Autodesk Inventor part; units mm, degrees
ref_plane "YZ Plane" through (0, 0, 0) normal (1, 0, 0) x (0, 1, 0)
ref_plane "XZ Plane" through (0, 0, 0) normal (0, 1, 0) x (-1, 0, 0)
ref_plane "XY Plane" through (0, 0, 0) normal (0, 0, 1) x (1, 0, 0)
sketch "Sketch1" plane through (0, 0, 0) normal (0, 0, 1) x (1, 0, 0)
  line L0 (0, 0) -> (170, 0)
  line L1 (170, 0) -> (170, 170)
  line L2 (170, 170) -> (0, 170)
  line L3 (0, 170) -> (0, 0)
  dimension "d0" = 170
  dimension "d1" = 170
extrude "Extrusion1" add sketch "Sketch1" along normal blind 2
sketch "Sketch2" plane through (0, 0, 2) normal (0, 0, 1) x (1, 0, 0)
  line L0 (170, 170) -> (0, 170)
  line L1 (0, 170) -> (0, 0)
  line L2 (0, 170) -> (0, 159.84) construction
  line L3 (0, 159.84) -> (6.35, 159.84) construction
  line L4 (6.35, 170) -> (163.83, 170) construction
  line L5 (163.83, 170) -> (163.83, 136.98) construction
  line L6 (6.35, 159.84) -> (6.35, 4.9) construction
  line L7 (6.35, 4.9) -> (163.83, 4.9) construction
  circle A0 centre (6.35, 159.84) radius 1.98
  circle A1 centre (163.83, 136.98) radius 1.98
  circle A2 centre (6.35, 4.9) radius 1.98
  circle A3 centre (163.83, 4.9) radius 1.98
  dimension "d4" = 10.16
  dimension "d5" = 6.35
  dimension "d6" = 157.48
  dimension "d7" = 33.02
  dimension "d8" = 154.94
  dimension "d9" = 3.96
  dimension "d10" = 3.96
  dimension "d11" = 3.96
  dimension "d12" = 3.96
extrude "Extrusion2" cut sketch "Sketch2" against normal blind 2
sketch "Sketch3" plane through (0, 0, 2) normal (0, 0, 1) x (1, 0, 0)
  line L0 (14.2327, 124.8626) -> (6.35, 124.8626)
  line L1 (6.35, 124.8626) -> (6.35, 41.7782)
  line L2 (6.35, 41.7782) -> (14.2327, 41.7782)
  line L3 (14.2327, 41.7782) -> (14.2327, 124.8626)
extrude "Extrusion3" add sketch "Sketch3" along normal blind 2
sketch "Sketch4" plane through (0, 0, 4) normal (0, 0, 1) x (1, 0, 0)
  line L0 (14.2327, 124.8626) -> (6.35, 124.8626)
  line L1 (6.35, 124.8626) -> (6.35, 41.7782)
  line L2 (6.35, 41.7782) -> (14.2327, 41.7782)
  line L3 (14.2327, 41.7782) -> (14.2327, 124.8626)
  line L4 (12.3491, 93.2345) -> (12.3491, 74.2867) construction
  line L5 (12.3491, 74.2867) -> (8.2093, 74.2867) construction
  line L6 (8.2093, 74.2867) -> (8.2093, 93.2345) construction
  line L7 (8.2093, 93.2345) -> (12.3491, 93.2345) construction
  point P0 (0, 0)
sketch "Sketch5" plane through (0, 0, 2) normal (0, 0, 1) x (1, 0, 0)
  line L0 (170, 170) -> (0, 170)
  line L1 (17.1297, 170) -> (152.7432, 170)
  line L2 (152.7432, 170) -> (152.7432, 149.8199)
  line L3 (152.7432, 149.8199) -> (17.1297, 149.8199)
  line L4 (17.1297, 149.8199) -> (17.1297, 170)
extrude "Extrusion4" add sketch "Sketch5" along normal blind 2
sketch "Sketch6" plane through (0, 0, 4) normal (0, 0, 1) x (1, 0, 0)
  line L0 (17.1297, 170) -> (17.1297, 149.8199)
  line L1 (17.1297, 149.8199) -> (152.7432, 149.8199)
  line L2 (152.7432, 149.8199) -> (152.7432, 170)
  line L3 (152.7432, 170) -> (17.1297, 170)
  line L4 (74.7193, 163.8007) -> (99.6305, 163.8007) construction
  line L5 (99.6305, 163.8007) -> (99.6305, 158.8439) construction
  line L6 (99.6305, 158.8439) -> (74.7193, 158.8439) construction
  line L7 (74.7193, 158.8439) -> (74.7193, 163.8007) construction
  point P0 (0, 0)
properties part number "mini itx motherboard"
Part model, mm, in its own coordinate system. Round coordinates to 2 decimals unless told otherwise and drop trailing zeros. Loops run counter-clockwise (first coordinate to the right, second up) from the corner with the lowest first, then second, coordinate; pieces in that order, holes last.
Item 1: Cut at B-B, the plane x = 163.83. Give the cut face in (y, z).
Item 2: Cut at C-C, the plane z = 2.8. Give the cut face in (x, y).
Item 3: Cut at A-A, the plane y = 4.9. Give the cut face in (x, z), then the cut area to 3 significant figures.
Item 4: Drop flat-ended pins along their axis: P1, Ø2, axis at y = 72, z = 2.5, coming from the +X side; P2, Ø2, axis at x = 52, z = 3.5, coming from the -Y side; P3, Ø1.6, axis at x = 11.5, z = 3.5, coming from the -Y side; P4, Ø5, axis at x = 163.83, y = 4.9, coming from the +Z side. Give the stop position or say it passes through.
Item 5: Cut at D-D, the plane y = 159.84. Give the cut face in (x, z), then the cut area to 3 significant figures.
Item 6: Mould opens along Y. For faces 1 (the face through (84, 86, 0)), 2 (the face through (86, 170, 2)), 3 (the face through (165.66, 136.22, 1.01)) say: +Y half, -Y half, draft (parallel to the pull), parting line (faces both ways), or undercut.
Item 7: Drill centre lines: line 1 (Y direction, x = 6.35, z = 1.65); line 2 (Y direction, x = 163.83, z = 1.2); line 3 (X direction, y = 159.84, z = 1.5). Where is each one in solid material? Low to high.
A:
1. outline: (0, 0) - (2.92, 0) - (2.92, 2) - (0, 2) - close; (6.88, 0) - (135, 0) - (135, 2) - (6.88, 2) - close; (138.96, 0) - (170, 0) - (170, 2) - (138.96, 2) - close
2. outline: (6.35, 41.78) - (14.23, 41.78) - (14.23, 124.86) - (6.35, 124.86) - close; (17.13, 149.82) - (152.74, 149.82) - (152.74, 170) - (17.13, 170) - close
3. outline: (0, 0) - (4.37, 0) - (4.37, 2) - (0, 2) - close; (8.33, 0) - (161.85, 0) - (161.85, 2) - (8.33, 2) - close; (165.81, 0) - (170, 0) - (170, 2) - (165.81, 2) - close
3. area: 324 mm2
4. P1: stops at x = 170
4. P2: stops at y = 149.82
4. P3: stops at y = 41.78
4. P4: stops at z = 2
5. outline: (0, 0) - (4.37, 0) - (4.37, 2) - (0, 2) - close; (8.33, 0) - (170, 0) - (170, 2) - (152.74, 2) - (152.74, 4) - (17.13, 4) - (17.13, 2) - (8.33, 2) - close
5. area: 603 mm2
6. face 1: draft
6. face 2: +Y half
6. face 3: undercut
7. line 1: y = 0 to 2.92, 6.88 to 157.86, 161.82 to 170
7. line 2: y = 0 to 2.92, 6.88 to 135, 138.96 to 170
7. line 3: x = 0 to 4.37, 8.33 to 170
